```python
from build123d import *

# Parameters (mm, degrees)
F3_DEPTH       = 3.81
F4_R           = 3.2639
F5_DEPTH       = 22.352
F6_R           = 1.9939
F7_DEPTH       = 4.826
F8_R           = 1.5875
F9_DEPTH       = 2.159
F10_W          = 9.4488
F10_H          = 4.5085
F11_DEPTH      = 25.4
F12_W          = 4.064
F12_H          = 3.81
F13_DEPTH      = 9.4752
F13_DEPTH_BACK = 9.4752


with BuildPart() as f1:
    # F0 (on Front) → F1 (revolve)
    with BuildSketch(Plane.XZ):
        Polygon((-27.305, 2.413), (-27.305, 0), (27.305, 0), (27.305, 9.4742), (23.495, 9.4742), (23.495, 4.5085), (-5.334, 4.5085), (-5.334, 3.4925), (-10.795, 3.4925), (-10.795, 2.413), align=None)
    revolve(axis=Axis((0, 0, 0), (1, 0, 0)))

    # F2 (on face) → F3 (cut, through all)
    with BuildSketch(Plane.YZ.offset(27.305)):
        with BuildLine():
            ThreePointArc((-2.0352498271, 9.253011606), (-7.3838617793, 5.9362488883), (-9.4742, 0))
            Line((-9.4742, 0), (-6.35, 0))
            Line((-6.35, 0), (-2.0352498271, 9.253011606))
        make_face()
        with BuildLine():
            Line((6.35, 0), (9.4742, 0))
            ThreePointArc((9.4742, 0), (7.3838617793, 5.9362488883), (2.0352498271, 9.253011606))
            Line((2.0352498271, 9.253011606), (6.35, 0))
        make_face()
    extrude(amount=-F3_DEPTH, mode=Mode.SUBTRACT)

    # F4 (on face) → F5 (cut)
    with BuildSketch(Plane.YZ.offset(27.305)):
        Circle(F4_R)
    extrude(amount=-F5_DEPTH, mode=Mode.SUBTRACT)

    # F6 (on face) → F7 (join)
    with BuildSketch(Plane.YZ.offset(27.305)):
        with Locations((0, 6.9342)):
            Circle(F6_R)
    extrude(amount=F7_DEPTH)

    # F8 (on face) → F9 (join)
    with BuildSketch(Plane.YZ.offset(32.131)):
        with Locations((0, 6.9342)):
            Circle(F8_R)
    extrude(amount=F9_DEPTH)

    # F10 (on Top) → F11 (cut)
    with BuildSketch(Plane.XY):
        with Locations((11.9126, 2.25425)):
            Rectangle(F10_W, F10_H)
    extrude(amount=F11_DEPTH, mode=Mode.SUBTRACT)

    # F12 (on Top) → F13 (cut, two sides)
    with BuildSketch(Plane.XY) as f13_sk:
        with Locations((-8.763, -4.445)):
            Rectangle(F12_W, F12_H)
        with Locations((-8.763, 4.445)):
            Rectangle(F12_W, F12_H)
    extrude(amount=-F13_DEPTH, mode=Mode.SUBTRACT)
    extrude(f13_sk.sketch, amount=F13_DEPTH_BACK, mode=Mode.SUBTRACT)


solid = f1.part
```
Read the model definition and answer for the solid it produces. Units are mm, in the model's axes. A direction names the side the tool comes from. Coordinates: 2 decimals unless noted, no trailing zeros. Write each loop counter-clockwise with the first axis right and the second up, starting at its lowest first coordinate (ties: lowest second). Pieces come first, ordered by that corner, then holes. Notation, with made-up numbers: (-18, 57) -> (20, 57) arc R31 cw to (20, 96) -> close; hole circle Ø4 at (33.5, 48). An arc over 180 degrees is marked (long way). Return JSON: item names as keys, results as strings.
1. A tool of negligible diameter and unlimited length cuts with its end or side. For faces 1 (the face through (16.637, 2, 3)), 2 (the face through (29.68, -0.26, 8.91)), 3 (the face through (25, 8, 0)), 4 (the face through (-19.166, 1.468, -1.915)), 5 (the face through (-9, -2.54, 0)), from which of +Z, -Z, +X, -X, +Y, -Y can it reach the whole face along a straight path? Write none if from no direction.
Found:
{"face 1": "+Z, +Y", "face 2": "+X", "face 3": "+Z, +X, -X, +Y", "face 4": "-X", "face 5": "+Z, -Z, -X, -Y"}
2. Determine the mould class of faces 6 (the face through (34.29, 0, 7)), 7 (the face through (8.88, -3.05, -3.32)), 8 (the face through (16.285, -2.59, -1.986)), 9 (the face through (4.953, 0, 0)) for opening direction Y: pulls with the +Y half, pulls with the -Y half, needs draft (parallel to the pull), parting line crosses it, or undercut.
Found:
{"face 6": "needs draft", "face 7": "parting line crosses it", "face 8": "undercut", "face 9": "undercut"}
3. Each of these flat-tipped pins is pushed along its axis until it touches: P1, Ø5.5, axis at y = -4.5, z = 1.5, coming from the +X side (3 decimals); P2, Ø6, axis at y = 0, z = 0, coming from the +X side; P3, Ø5, axis at y = 7, z = 7, coming from the -X side; P4, Ø2.5, axis at x = 25, y = 8.5, coming from the +Z side. Where does it stop, or does it pass through?
Found:
{"P1": "x = 27.305", "P2": "x = 4.95", "P3": "through", "P4": "z = 0"}
4. A cutting plane is placed at B-B (x = -3). Determine the outline of the cut face in (y, z).
Found:
{"outline": "circle Ø9.02 at (0, 0)"}
5. A cutting plane is placed at A-A (x = 19.5). Determine the outline of the cut face in (y, z).
Found:
{"outline": "circle Ø9.02 at (0, 0); hole circle Ø6.53 at (0, 0)"}
6. Find the intervals of material crossed by line 1 along X through (y, z) = (-5, -2) (3 decimals); line 2 along X through (y, z) = (1.5, 4) (3 decimals); line 3 along X through (y, z) = (1, -1.5) (3 decimals), in increasing order. Write a range as from..to.
Found:
{"line 1": "23.495..27.305", "line 2": "-5.334..7.188, 16.637..27.305", "line 3": "-27.305..4.953"}
7. A cutting plane is placed at D-D (z = -8.5). Determine the outline of the cut face in (x, y) (3 decimals), and give its area (3 significant figures).
Found:
{"outline": "(23.495, -4.185) -> (27.305, -4.185) -> (27.305, 4.185) -> (23.495, 4.185) -> close", "area": "31.9 mm2"}
8. A cutting plane is placed at C-C (y = -1). Determine the outline of the cut face in (x, z) (3 decimals).
Found:
{"outline": "(-27.305, -2.196) -> (-10.795, -2.196) -> (-10.795, -3.346) -> (-5.334, -3.346) -> (-5.334, -4.396) -> (23.495, -4.396) -> (23.495, -9.421) -> (27.305, -9.421) -> (27.305, -3.107) -> (4.953, -3.107) -> (4.953, 3.107) -> (27.305, 3.107) -> (27.305, 5.209) -> (32.131, 5.209) -> (32.131, 5.701) -> (34.29, 5.701) -> (34.29, 8.167) -> (32.131, 8.167) -> (32.131, 8.659) -> (27.305, 8.659) -> (27.305, 9.421) -> (23.495, 9.421) -> (23.495, 4.396) -> (-5.334, 4.396) -> (-5.334, 3.346) -> (-10.795, 3.346) -> (-10.795, 2.196) -> (-27.305, 2.196) -> close"}
